Geometry check sheet. Reference: the model listing, model coordinates, mm. A direction names the side the tool comes from. Give positions to 0.01 mm unless a question says otherwise; leave off trailing zeros. Loops run counter-clockwise (first coordinate to the right, second up) from the corner with the lowest first, then second, coordinate; pieces in that order, holes last. Notation, with made-up numbers: (69, 24.25) -> (107, 24.25) arc R24 ccw to (107, 40.25) -> close; hole circle Ø1 at (-38, 6.25). An arc over 180 degrees is marked (long way). Write item = value, one per line.
Autodesk Fusion 360 part; units mm, degrees
sketch "Skizze1" plane through (0, 0, 0) normal (0, 1, 0) x (1, 0, 0)
  line L0 (0, 0) -> (30, 0)
  line L1 (30, 0) -> (30, 66)
  line L2 (30, 66) -> (0, 66)
  line L3 (0, 66) -> (0, 0)
  dimension "d5" = 30
  dimension "d6" = 66
extrude "Extrusion2" add sketch "Skizze1" along normal blind 42.2
sketch "Skizze2" plane through (0, 42.2, 0) normal (0, 1, 0) x (-1, 0, 0)
  line L0 (0, -66) -> (0, 0)
  line L1 (0, 0) -> (-30, 0)
  line L2 (-30, 0) -> (-30, -66)
  line L3 (-30, -66) -> (0, -66)
  line L4 (0, -74.5) -> (-30, -74.5)
  line L5 (-30, -74.5) -> (-30, 8.5)
  line L6 (-30, 8.5) -> (0, 8.5)
  line L7 (0, 8.5) -> (0, -74.5)
  line L8 (-30, -66) -> (0, 0) construction
  line L9 (0, -74.5) -> (-30, 8.5) construction
  line L10 (-15, -33) -> (-15, -70.5) construction
  line L11 (-15, -70.5) -> (-6, -70.5) construction
  circle A0 centre (-6, -70.5) radius 2.25
  circle A1 centre (-24, -70.5) radius 2.25
  circle A2 centre (-6, 4.5) radius 2.25
  circle A3 centre (-24, 4.5) radius 2.25
  line L12 (-4.6, -74.5) -> (-7.4, -74.5)
  line L13 (-7.4, -74.5) -> (-7.4, -71.5)
  line L14 (-7.4, -71.5) -> (-4.6, -71.5)
  line L15 (-4.6, -71.5) -> (-4.6, -74.5)
  line L16 (-6, -71.5) -> (-6, -70.5) construction
  line L17 (-25.4, -74.5) -> (-25.4, -71.5)
  line L18 (-22.6, -74.5) -> (-25.4, -74.5)
  line L19 (-22.6, -71.5) -> (-22.6, -74.5)
  line L20 (-25.4, -71.5) -> (-22.6, -71.5)
  line L21 (-7.4, 5.5) -> (-7.4, 8.5)
  line L22 (-4.6, 5.5) -> (-7.4, 5.5)
  line L23 (-4.6, 8.5) -> (-4.6, 5.5)
  line L24 (-7.4, 8.5) -> (-4.6, 8.5)
  line L25 (-25.4, 5.5) -> (-25.4, 8.5)
  line L26 (-22.6, 5.5) -> (-25.4, 5.5)
  line L27 (-22.6, 8.5) -> (-22.6, 5.5)
  line L28 (-25.4, 8.5) -> (-22.6, 8.5)
  point P0 (-15, -33)
  dimension "d9" = 30
  dimension "d10" = 83
  dimension "d13" = 9
  dimension "d14" = 37.5
  dimension "d15" = 4.5
  dimension "d18" = -18
  dimension "d19" = 75
  dimension "d20" = 2.8
  dimension "d21" = 3
  dimension "d24" = -18
  dimension "d25" = 80
extrude "Extrusion3" add sketch "Skizze2" along normal blind 4 contours L0 L1 L2 L3 L5 L7 | L3 L4 L5 L7 A0 A1 L13 L15 L17 L19 | L1 L5 L6 L7 A2 A3 L21 L23 L25 L27
sketch "Skizze3" plane through (0, 46.2, 0) normal (0, 1, 0) x (-1, 0, 0)
  line L0 (-7.4, 6.2614) -> (-7.4, 8.5)
  line L1 (-7.4, 8.5) -> (-22.6, 8.5)
  line L2 (-22.6, 8.5) -> (-22.6, 6.2614)
  arc A0 (-25.4, 6.2614) -> (-22.6, 6.2614) centre (-24, 4.5) ccw
  line L3 (-25.4, 6.2614) -> (-25.4, 8.5)
  line L4 (-25.4, 8.5) -> (-30, 8.5)
  line L5 (-30, 8.5) -> (-30, -74.5)
  line L6 (-30, -74.5) -> (-25.4, -74.5)
  line L7 (-25.4, -74.5) -> (-25.4, -72.2614)
  arc A1 (-22.6, -72.2614) -> (-25.4, -72.2614) centre (-24, -70.5) ccw
  line L8 (-22.6, -72.2614) -> (-22.6, -74.5)
  line L9 (-22.6, -74.5) -> (-7.4, -74.5)
  line L10 (-7.4, -74.5) -> (-7.4, -72.2614)
  arc A2 (-4.6, -72.2614) -> (-7.4, -72.2614) centre (-6, -70.5) ccw
  line L11 (-4.6, -72.2614) -> (-4.6, -74.5)
  line L12 (-4.6, -74.5) -> (0, -74.5)
  line L13 (0, -74.5) -> (0, 8.5)
  line L14 (0, 8.5) -> (-4.6, 8.5)
  line L15 (-4.6, 8.5) -> (-4.6, 6.2614)
  arc A3 (-7.4, 6.2614) -> (-4.6, 6.2614) centre (-6, 4.5) ccw
  line L16 (-30, -66) -> (0, -66)
  line L17 (0, 0) -> (-30, 0)
  line L18 (0, -66) -> (-30, -66)
  line L19 (-30, 0) -> (0, 0)
extrude "Extrusion4" add sketch "Skizze3" along normal blind 3.5 contours L5 L13 L16 L17 L18 L19
fillet "Abrundung1" radius 2 4 edges at (30, 44.2, -74.5) (0, 44.2, -74.5) (30, 44.2, 8.5) (0, 44.2, 8.5)
sketch "Skizze4" plane through (0, 49.7, 0) normal (0, 1, 0) x (-1, 0, 0)
  line L0 (0, -66) -> (0, 0)
  line L1 (0, 0) -> (-30, 0)
  line L2 (-30, 0) -> (-30, -66)
  line L3 (-30, -66) -> (0, -66)
  line L4 (-30, -66) -> (0, -66)
  line L5 (0, -66) -> (0, 0)
  line L6 (-30, 0) -> (-30, -66)
  line L7 (0, 0) -> (-30, 0)
  line L8 (0, -52.3857) -> (-7.8134, -52.3857)
  line L9 (-30, -55.8819) -> (-20.9697, -55.8819)
  arc A0 (-20.9697, -55.8819) -> (-7.8134, -52.3857) centre (-14.8561, -52.3857) ccw
  line L10 (-30, -66) -> (0, -66)
  line L11 (0, -66) -> (0, 0)
  line L12 (-30, 0) -> (-30, -66)
  dimension "d31" = 13.6143
  dimension "d32" = 10.1181
  dimension "d33" = 7.8134
  dimension "d35" = 9.0303
extrude "Extrusion5" add sketch "Skizze4" along normal blind 6.507 contours L0 L1 L2 L5 L6 L7 L8 L9 A0 L11 L12
sketch "Skizze5" plane through (0, 56.207, 0) normal (0, 1, 0) x (-1, 0, 0)
  line L0 (0, -52.3857) -> (0, 0)
  line L1 (0, 0) -> (-30, 0)
  line L2 (-30, 0) -> (-30, -55.8819)
  line L3 (-30, -55.8819) -> (-20.9697, -55.8819)
  arc A0 (-20.9697, -55.8819) -> (-7.8134, -52.3857) centre (-14.8561, -52.3857) ccw
  line L4 (-7.8134, -52.3857) -> (0, -52.3857)
  circle A1 centre (-15, -15) radius 9.4153
  line L5 (-30, 0) -> (-30, -66)
  line L6 (0, 0) -> (-30, 0)
  dimension "d39" = 15
  dimension "d40" = 15
  dimension "d41" = 18.8307
extrude "Extrusion6" add sketch "Skizze5" along normal blind 4.5 contours A1
sketch "Skizze6" plane through (0, 60.707, 0) normal (0, 1, 0) x (-1, 0, 0)
  circle A0 centre (-15, -15) radius 9.4153
  circle A1 centre (-15, -15) radius 9.4153
  circle A2 centre (-15, -15) radius 3.315
  dimension "d45" = 6.63
extrude "Extrusion7" add sketch "Skizze6" along normal blind 6 contours A2
fillet "Abrundung3" radius 2 1 edges at (23.7782, 60.707, -18.4047)
fillet "Abrundung2" radius 1 7 edges at (13.0473, 56.207, -59.1921) (3.9067, 56.207, -52.3857) (25.4848, 56.207, -55.8819) (15, 49.7, -66) (15, 56.207, 0) (30, 56.207, -27.9409) (0, 56.207, -26.1929)
equation "d13 = ( 18 / 2 ) * 1 mm"
equation "d14 = ( 75 / 2 ) * 1 mm"
Item 1: Section check A-A, the plane z = 4.5. Record the cut outline in (x, y).
Answer:
outline = (0, 42.2) -> (3.75, 42.2) -> (3.75, 46.2) -> (0, 46.2) -> close; (8.25, 42.2) -> (21.75, 42.2) -> (21.75, 46.2) -> (8.25, 46.2) -> close; (26.25, 42.2) -> (30, 42.2) -> (30, 46.2) -> (26.25, 46.2) -> close
Item 2: Section check D-D, the plane y = 54. Record the cut outline in (x, z), plus the area to 3 significant figures.
Answer:
outline = (0, -52.39) -> (7.81, -52.39) arc R7.04 ccw to (20.97, -55.88) -> (30, -55.88) -> (30, 0) -> (0, 0) -> close
area = 1,680 mm^2
Item 3: Draft check along Z on faces 6 (the cylindrical face through (24.08, 44.17, -68.25)), 7 (the flat face through (15, 56.207, -29)), 8 (the flat face through (15, 44, -74.5)). Enter one of: +Z half, -Z half, draft (parallel to the pull), parting line (faces both ways), or undercut.
Answer:
face_6 = undercut
face_7 = draft
face_8 = -Z half
Item 4: Section check B-B, the plane y = 45. Record the cut outline in (x, z).
Answer:
outline = (0, -72.5) arc R2 ccw to (2, -74.5) -> (4.6, -74.5) -> (4.6, -72.26) arc R2.25 cw (long way) to (7.4, -72.26) -> (7.4, -74.5) -> (22.6, -74.5) -> (22.6, -72.26) arc R2.25 cw (long way) to (25.4, -72.26) -> (25.4, -74.5) -> (28, -74.5) arc R2 ccw to (30, -72.5) -> (30, 6.5) arc R2 ccw to (28, 8.5) -> (25.4, 8.5) -> (25.4, 6.26) arc R2.25 cw (long way) to (22.6, 6.26) -> (22.6, 8.5) -> (7.4, 8.5) -> (7.4, 6.26) arc R2.25 cw (long way) to (4.6, 6.26) -> (4.6, 8.5) -> (2, 8.5) arc R2 ccw to (0, 6.5) -> close
Item 5: Tool access check on faces 1 (the flat face through (7.4, 44, -73)), 2 (the flat face through (15, 49.7, -60)), 3 (the flat face through (15, 21, -66)), 4 (the flat face through (15, 46.2, 4)), 5 (the flat face through (4.6, 44, 7)). Record the directions out of +Z, -Z, +X, -X, +Y, -Y that give a thin tool (end or side, any length) a straight path to the whole face; none if there is none.
Answer:
face_1 = -Z, +Y, -Y
face_2 = -Z, +Y
face_3 = -Z, +X, -X, -Y
face_4 = +Z, +X, -X, +Y
face_5 = +Z, +Y, -Y
Item 6: Section check C-C, the plane z = -33. Record the cut outline in (x, y), plus the area to 3 significant figures.
Answer:
outline = (0, 0) -> (30, 0) -> (30, 55.21) arc R1 ccw to (29, 56.21) -> (1, 56.21) arc R1 ccw to (0, 55.21) -> close
area = 1,690 mm^2
Item 7: Thickness scan on L1, parallel to X at y = 44.6, z = 4.5; L2, parallel to Z at x = 24, y = 43.25; L3, parallel to Z at x = 20, y = 31. Record the ranges inside material, lowest first. Write a range as [from, to].
Answer:
L1 = [0, 3.75], [8.25, 21.75], [26.25, 30]
L2 = [-68.25, 2.25]
L3 = [-66, 0]
Item 8: Gauge pin test, flat ends, axial feed: pin 1 (1 mm diameter, centred on x = 20, y = 21, fed in from -Z); pin 2 (9.5 mm diameter, centred on x = 22.5, z = 2.5, fed in from +Y); pin 3 (10 mm diameter, centred on x = 21.5, y = 50.5, fed in from +Z); pin 4 (6 mm diameter, centred on x = 6, z = -70.5, fed in from +Y). Record the tip position at first contact, or that the pin passes through.
Answer:
pin_1 = -66
pin_2 = 56.21
pin_3 = 8.5
pin_4 = 46.2
